Check sheet for the modelled part. Datum: model origin and axes. Units: mm. Face numbers are marked on the shaded views. A direction names the side the tool comes from. Coordinates: 2 decimals unless noted, no trailing zeros. Write each loop counter-clockwise with the first axis right and the second up, starting at its lowest first coordinate (ties: lowest second). Pieces come first, ordered by that corner, then holes. Notation, with made-up numbers: (6, 36.5) -> (52, 36.5) arc R12 cw to (52, 47.5) -> close; hole circle Ø4 at (14, 68.5). An arc over 180 degrees is marked (long way). One line per item, written item: value. Start each with the question number.
1) Sectioned sample at A-A on z = 6. Enter the section's corners in (x, y), plus the area to 3 significant figures.
2) Gauge pin test, flat ends, axial feed: P1, Ø6, axis at x = -19.5, y = -2, coming from the -Z side; P2, Ø17.5, axis at x = 15, y = -12, coming from the -Z side; P3, Ø10, axis at x = -13.5, y = -4, coming from the +Z side; P4, Ø1, axis at y = 14.5, z = 13, coming from the -X side. Record the tip position at first contact, or that the pin passes through.
3) Draft check along X on the marked faces 1, 2 and 3. Enter one of: +X half, -X half, draft (parallel to the pull), parting line (faces both ways), or undercut.
4) Sectioned sample at C-C on x = -15. Enter the section's corners in (y, z), plus the area to 3 significant figures.
5) Sectioned sample at B-B on y = -12. Enter the section's corners in (x, z), plus the area to 3 significant figures.
6) Set-up check for the marked faces 4 and 5: record each of +Z, -Z, +X, -X, +Y, -Y from which the full face is reachable in a straight line by a thin tool's end or side.
7) Sectioned sample at D-D on y = 21. Enter the section's corners in (x, z).
8) Scan lines: line 1 along Y through (x, z) = (-15, 6); line 2 along X through (y, z) = (-5.5, 1.75); line 3 along X through (y, z) = (-18, 1.5). Record each from-to range of solid material in increasing order. Write a range as [from, to].
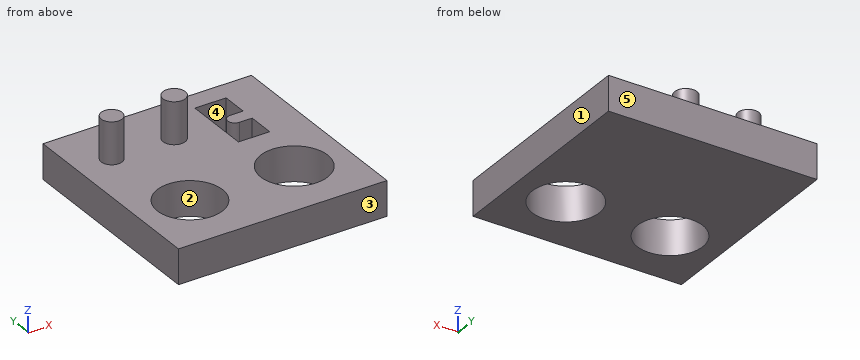
```python
from build123d import *

# Parameters (mm, degrees)
F0_W     = 60
F0_H     = 60
F1_DEPTH = 10
F2_R     = 3
F2_R_2   = 3.2
F3_DEPTH = 12
F4_R     = 9.4
F4_R_2   = 9.65
F5_DEPTH = 10
F7_DEPTH = 9.55


with BuildPart() as f1:
    # F0 (on Top) → F1 (new body)
    with BuildSketch(Plane.XY):
        Rectangle(F0_W, F0_H)
    extrude(amount=F1_DEPTH)

    # F2 (on face) → F3 (join)
    with BuildSketch(Plane.XY.offset(10)):
        with Locations((-20, 15)):
            Circle(F2_R)
        with Locations((-2, 15)):
            Circle(F2_R_2)
    extrude(amount=F3_DEPTH)

    # F4 (on face) → F5 (cut, through all)
    with BuildSketch(Plane.XY.offset(10)):
        with Locations((-15, -12)):
            Circle(F4_R)
        with Locations((15, -12)):
            Circle(F4_R_2)
    extrude(amount=-F5_DEPTH, mode=Mode.SUBTRACT)

    # F6 (on face) → F7 (cut)
    with BuildSketch(Plane.XY.offset(10)):
        with BuildLine():
            Line((19, 24.3), (10, 24.3))
            Line((10, 24.3), (10, 5))
            Line((10, 5), (19, 5))
            Line((19, 5), (19, 12.75))
            Line((19, 12.75), (15.3, 12.75))
            ThreePointArc((15.3, 12.75), (13.3, 14.75), (15.3, 16.75))
            Line((15.3, 16.75), (19, 16.75))
            Line((19, 16.75), (19, 24.3))
        make_face()
    extrude(amount=-F7_DEPTH, mode=Mode.SUBTRACT)


solid = f1.part
```
Answers:
1. outline: (-30, -30) -> (30, -30) -> (30, 30) -> (-30, 30) -> close; hole circle Ø18.8 at (-15, -12); hole circle Ø19.3 at (15, -12); hole (10, 5) -> (19, 5) -> (19, 12.75) -> (15.3, 12.75) arc R2 cw to (15.3, 16.75) -> (19, 16.75) -> (19, 24.3) -> (10, 24.3) -> close
1. area: 2,880 mm2
2. P1: stops at z = 0
2. P2: passes through
2. P3: stops at z = 10
2. P4: stops at x = -23
3. face 1: +X half
3. face 2: undercut
3. face 3: draft
4. outline: (-30, 0) -> (-21.4, 0) -> (-21.4, 10) -> (-30, 10) -> close; (-2.6, 0) -> (30, 0) -> (30, 10) -> (-2.6, 10) -> close
4. area: 412 mm2
5. outline: (-30, 0) -> (-24.4, 0) -> (-24.4, 10) -> (-30, 10) -> close; (-5.6, 0) -> (5.35, 0) -> (5.35, 10) -> (-5.6, 10) -> close; (24.65, 0) -> (30, 0) -> (30, 10) -> (24.65, 10) -> close
5. area: 219 mm2
6. face 4: +Z
6. face 5: +Z, -Z, +X, -X, +Y
7. outline: (-30, 0) -> (30, 0) -> (30, 10) -> (19, 10) -> (19, 0.45) -> (10, 0.45) -> (10, 10) -> (-30, 10) -> close
8. line 1: y = [-30, -21.4], [-2.6, 30]
8. line 2: x = [-30, -21.79], [-8.21, 7.87], [22.13, 30]
8. line 3: x = [-30, -22.24], [-7.76, 7.44], [22.56, 30]
